Autodesk Inventor part; units mm, degrees
ref_plane "YZ Plane" through (0, 0, 0) normal (1, 0, 0) x (0, 1, 0)
ref_plane "XZ Plane" through (0, 0, 0) normal (0, 1, 0) x (-1, 0, 0)
ref_plane "XY Plane" through (0, 0, 0) normal (0, 0, 1) x (1, 0, 0)
sketch "Sketch1" plane through (0, 0, 0) normal (0, 0, 1) x (1, 0, 0)
  line L0 (-26, 13) -> (26, 13)
  line L1 (26, -13) -> (-26, -13)
  line L2 (-26, 13) -> (26, -13) construction
  line L3 (26, 13) -> (-26, -13) construction
  line L4 (-41.6, 15.6) -> (41.6, 15.6)
  line L5 (41.6, 15.6) -> (41.6, -15.6)
  line L6 (41.6, -15.6) -> (-41.6, -15.6)
  line L7 (-41.6, -15.6) -> (-41.6, 15.6)
  line L8 (-41.6, 15.6) -> (41.6, -15.6) construction
  line L9 (41.6, 15.6) -> (-41.6, -15.6) construction
  line L10 (-26, 1.3) -> (-35.75, 1.3)
  line L11 (-35.75, 1.3) -> (-35.75, -1.3)
  line L12 (-35.75, -1.3) -> (-26, -1.3)
  line L13 (26, 1.3) -> (35.75, 1.3)
  line L14 (35.75, 1.3) -> (35.75, -1.3)
  line L15 (35.75, -1.3) -> (26, -1.3)
  line L16 (-26, 1.3) -> (-26, 13)
  line L17 (-26, -13) -> (-26, -1.3)
  line L18 (26, -1.3) -> (26, -13)
  line L19 (26, 1.3) -> (26, 13)
  point P0 (0, 0)
  point P1 (-35.75, 0)
  point P2 (0, 0)
  dimension "CInt" = 52
  dimension "LInt" = 26
  dimension "Cext" = 83.2
  dimension "Lext" = 31.2
  dimension "Cpeq" = 9.75
  dimension "Lpeq" = 2.6
  dimension "d10" = 9.75
  dimension "d11" = 2.6
extrude "Extrusion1" add sketch "Sketch1" along normal mid plane 6.5
sketch "Sketch8" plane through (0, 0, 3.25) normal (0, 0, 1) x (1, 0, 0)
  point P0 (0, 0)
hole "Hole1" at (-32.5, 6.5, 3.25) direction (0, 0, -1) diameter 6.5 end through all
pattern_linear "Rectangular Pattern1" count 2 spacing 13 along (0, -1, 0) of "Hole1"
hole "Hole2" at (32.5, 6.5, 3.25) direction (0, 0, -1) diameter 6.5 end through all
pattern_linear "Rectangular Pattern2" count 2 spacing 13 along (0, -1, 0) of "Hole2"
properties part number "DandoBom"
Part model, mm, in its own coordinate system. A direction names the side the tool comes from. Round coordinates to 2 decimals unless told otherwise and drop trailing zeros. Write each loop counter-clockwise with the first axis right and the second up, starting at its lowest first coordinate (ties: lowest second). Pieces come first, ordered by that corner, then holes.
Item 1: Which spindle directions (+Z, -Z, +X, -X, +Y, -Y) get a long thin tool onto all of the face, cutting with end or side? Do faces 4 (the flat face through (-31, 1.3, 0)), 5 (the flat face through (-1, 15.6, 0)). Say none if no direction does.
Results:
face 4: +Z, -Z
face 5: +Z, -Z, +X, -X, +Y
Item 2: Cut at A-A, the plane y = 11. Give the cut face in (x, z), plus the area to 3 significant figures.
Results:
outline: (-41.6, -3.25) - (-26, -3.25) - (-26, 3.25) - (-41.6, 3.25) - close; (26, -3.25) - (41.6, -3.25) - (41.6, 3.25) - (26, 3.25) - close
area: 203 mm2
Item 3: Probe L1, parallel to X at y = 6.5, z = 1.25; L2, parallel to Y at x = -32.5, z = 2.25; L3, parallel to Y at x = 30, z = 0. List the from-to ranges inside material, lowest first.
Results:
L1: x = -41.6 to -35.75, -29.25 to -26, 26 to 29.25, 35.75 to 41.6
L2: y = -15.6 to -9.75, -3.25 to -1.3, 1.3 to 3.25, 9.75 to 15.6
L3: y = -15.6 to -8.58, -4.42 to -1.3, 1.3 to 4.42, 8.58 to 15.6
Item 4: Cut at D-D, the plane x = 32.5. Give the cut face in (y, z), plus the area to 3 significant figures.
Results:
outline: (-15.6, -3.25) - (-9.75, -3.25) - (-9.75, 3.25) - (-15.6, 3.25) - close; (-3.25, -3.25) - (-1.3, -3.25) - (-1.3, 3.25) - (-3.25, 3.25) - close; (1.3, -3.25) - (3.25, -3.25) - (3.25, 3.25) - (1.3, 3.25) - close; (9.75, -3.25) - (15.6, -3.25) - (15.6, 3.25) - (9.75, 3.25) - close
area: 101 mm2
Item 5: Drop flat-ended pins along their axis: pin 1 Ø4 at (x, y) = (-32.5, 6.5) entering from +Z; pin 2 Ø7.5 at (x, y) = (32.5, -6.5) entering from -Z. Give the stop position or say it passes through.
Results:
pin 1: passes through
pin 2: stops at z = -3.25
Item 6: Cut at C-C, the plane z = 1.5. Give the cut face in (x, y).
Results:
outline: (-41.6, -15.6) - (41.6, -15.6) - (41.6, 15.6) - (-41.6, 15.6) - close; hole circle Ø6.5 at (-32.5, -6.5); hole (-35.75, -1.3) - (-26, -1.3) - (-26, -13) - (26, -13) - (26, -1.3) - (35.75, -1.3) - (35.75, 1.3) - (26, 1.3) - (26, 13) - (-26, 13) - (-26, 1.3) - (-35.75, 1.3) - close; hole circle Ø6.5 at (-32.5, 6.5); hole circle Ø6.5 at (32.5, -6.5); hole circle Ø6.5 at (32.5, 6.5)
Item 7: Cut at B-B, the plane x = 12.5. Give the cut face in (y, z), plus the area to 3 significant figures.
Results:
outline: (-15.6, -3.25) - (-13, -3.25) - (-13, 3.25) - (-15.6, 3.25) - close; (13, -3.25) - (15.6, -3.25) - (15.6, 3.25) - (13, 3.25) - close
area: 33.8 mm2
Item 8: Two-plate mould, pull along X, no slides. Class faces 1 (the flat face through (41.6, 0, 0)), 2 (the flat face through (1, -15.6, 0)), 3 (the flat face through (-26, 7, 0)): +X half, -X half, draft (parallel to the pull), parting line (faces both ways), or undercut.
Results:
face 1: +X half
face 2: draft
face 3: undercut
